Read the model definition and answer for the solid it produces. Units are mm, in the model's axes. A direction names the side the tool comes from. Coordinates: 2 decimals unless noted, no trailing zeros. Order: outer loops, then holes, each group sorted by start corner. A loop starts at its lowest first (then second) coordinate and runs counter-clockwise, first axis right, second up.
```python
from build123d import *

# Parameters (mm, degrees)
SKETCH1_W           = 228.6
SKETCH1_H           = 50.8
BOSS_EXTRUDE1_DEPTH = 5
SKETCH2_R           = 2.000000064
CUT_EXTRUDE1_DEPTH  = 118.194923098
SKETCH3_W           = 17.431165178
SKETCH3_H           = 100
BOSS_EXTRUDE2_DEPTH = 4
SKETCH4_W           = 12.7
SKETCH4_H           = 15
BOSS_EXTRUDE3_DEPTH = 6
CUT_EXTRUDE2_REACH  = 250.519
SKETCH5_R           = 2.000000064
SKETCH5_R_2         = 2
SKETCH6_R           = 3.5
CUT_EXTRUDE3_DEPTH  = 3
FILLET2_R           = 2.54


with BuildPart() as part:
    # Sketch1 → Boss-Extrude1 (new body)
    with BuildSketch(Plane.XY):
        Rectangle(SKETCH1_W, SKETCH1_H)
    extrude(amount=BOSS_EXTRUDE1_DEPTH)

    # Sketch2 → Cut-Extrude1 (cut, through all)
    with BuildSketch(Plane.XY.offset(5)):
        with Locations((-88.9, 0)):
            Circle(SKETCH2_R)
    extrude(amount=-CUT_EXTRUDE1_DEPTH, mode=Mode.SUBTRACT)

    # Sketch3 → Boss-Extrude2 (add)
    with BuildSketch(Plane(origin=(114.3, 0, 0), x_dir=(0, 0, -1), z_dir=(1, 0, 0))):
        with Locations((-2.5, -18.6)):
            Rectangle(SKETCH3_W, SKETCH3_H)
    extrude(amount=BOSS_EXTRUDE2_DEPTH)

    # Sketch4 → Boss-Extrude3 (add)
    with BuildSketch(Plane(origin=(118.3, 0, 0), x_dir=(0, 0, -1), z_dir=(1, 0, 0))):
        with Locations((-2.5, -44.840000008)):
            Rectangle(SKETCH4_W, SKETCH4_H)
    extrude(amount=BOSS_EXTRUDE3_DEPTH)

    # Sketch5 → Cut-Extrude2 (cut, up to next)
    with BuildSketch(Plane(origin=(124.3, 0, 0), x_dir=(0, 0, -1), z_dir=(1, 0, 0)), mode=Mode.PRIVATE) as cut_extrude2_sk1:
        with Locations((-2.5, -39.840000088)):
            Circle(SKETCH5_R)
    cut_extrude2_tool1 = extrude(cut_extrude2_sk1.sketch, amount=-CUT_EXTRUDE2_REACH, mode=Mode.PRIVATE) & part.part
    # Sketch5 → Cut-Extrude2 (cut, up to next)
    with BuildSketch(Plane(origin=(124.3, 0, 0), x_dir=(0, 0, -1), z_dir=(1, 0, 0)), mode=Mode.PRIVATE) as cut_extrude2_sk2:
        with Locations((-2.5, -49.840000088)):
            Circle(SKETCH5_R_2)
    cut_extrude2_tool2 = extrude(cut_extrude2_sk2.sketch, amount=-CUT_EXTRUDE2_REACH, mode=Mode.PRIVATE) & part.part
    add(cut_extrude2_tool1.solids().sort_by_distance((124.3, -39.84, 2.5))[0], mode=Mode.SUBTRACT)
    add(cut_extrude2_tool2.solids().sort_by_distance((124.3, -49.84, 2.5))[0], mode=Mode.SUBTRACT)

    # Sketch6 → Cut-Extrude3 (cut)
    with BuildSketch(Plane.ZY.offset(-114.3)):
        with Locations((2.5, -39.840000088)):
            Circle(SKETCH6_R)
        with Locations((2.5, -49.840000088)):
            Circle(SKETCH6_R)
    extrude(amount=-CUT_EXTRUDE3_DEPTH, mode=Mode.SUBTRACT)

    # Fillet2
    fillet2_edges = [part.edges().sort_by_distance(p)[0] for p in [
        (114.3, 0, 5),
        (114.3, 0, 0),
        (114.3, -25.4, 2.5),
        (114.3, 25.4, 2.5),
    ]]
    fillet(fillet2_edges, radius=FILLET2_R)


solid = part.part
```
1) A cutting plane is placed at B-B, the plane x = -83. Determine the outline of the cut face in (y, z).
A:
outline: (-25.4, 0) - (25.4, 0) - (25.4, 5) - (-25.4, 5) - close
2) Determine the mould class of faces 5 (the flat face through (118.3, -7, 3)), 6 (the flat face through (121, -45, 8.85)), 7 (the flat face through (117.3, -52, 2)) for opening direction Z: pulls with the +Z half, pulls with the -Z half, needs draft (parallel to the pull), parting line crosses it, or undercut.
A:
face 5: needs draft
face 6: pulls with the +Z half
face 7: undercut
3) Straight lines are drawn through the part: line 1 (Y direction, x = 121.75, z = 2.5); line 2 (Y direction, x = 115.9, z = 2.5); line 3 (X direction, y = 4, z = 1.5). For each, find the intervals that lie inside material, in ascending order.
A:
line 1: y = -52.34 to -51.84, -47.84 to -41.84, -37.84 to -37.34
line 2: y = -68.6 to -53.34, -46.34 to -43.34, -36.34 to 31.4
line 3: x = -114.3 to 118.3
4) Flat-ended cylindrical pins translate along their axes: pin 1 Ø4 at (x, y) = (89.5, -19) entering from +Z; pin 2 Ø1 at (x, z) = (-71.5, 6.5) entering from -Y; pin 3 Ø1.8 at (x, y) = (120, -42.5) entering from -Z; pin 4 Ø6.5 at (x, y) = (122.5, -42.5) entering from +Z. Find the tip coordinate at first contact, or state that the pin passes through.
A:
pin 1: stops at z = 5
pin 2: passes through
pin 3: stops at z = -3.85
pin 4: stops at z = 8.85
5) A cutting plane is placed at A-A, the plane y = -33.5. Determine the outline of the cut face in (x, z), and give its area (3 significant figures).
A:
outline: (114.3, -6.22) - (118.3, -6.22) - (118.3, 11.22) - (114.3, 11.22) - close
area: 69.7 mm2
6) Which of the six approach directions +Z, -Z, +X, -X, +Y, -Y give full straight-line access (tool end or side, diameter ignored) to faces 1 (the flat face through (121, -45, -3.85)), 2 (the flat face through (117.3, -40, 5)), 3 (the flat face through (121, -37.34, 3)), 4 (the flat face through (-3, -25.4, 2))?
A:
face 1: -Z, +X, +Y, -Y
face 2: -X
face 3: +Z, -Z, +X, +Y
face 4: +Z, -Z, -X, -Y
